```python
from build123d import *

# Parameters (mm, degrees)
BOSS_EXTRUDE1_DEPTH = 2.5
SKETCH3_R           = 4
CUT_EXTRUDE2_DEPTH  = 5


with BuildPart() as part:
    # Sketch1 → Boss-Extrude1 (new, symmetric)
    with BuildSketch(Plane(origin=(0, 0, 0), x_dir=(0, 1, 0), z_dir=(0, 0, 1))):
        Polygon((-56, 9.27), (-56, -9.27), (-50, -9.27), (-50, -12.741071429), (-50, -14.27), (-40, -14.27), (-40, -10.192857143), (-40, -9.27), (40, -9.27), (40, -10.192857143), (40, -14.27), (50, -14.27), (50, -9.27), (56, -9.27), (56, 9.27), (50, 9.27), (50, 14.27), (40, 14.27), (40, 9.27), (-40, 9.27), (-40, 10.192857143), (-40, 14.27), (-50, 14.27), (-50, 12.741071429), (-50, 9.27), align=None)
    extrude(amount=BOSS_EXTRUDE1_DEPTH, both=True)

    # Sketch3 → Cut-Extrude2 (cut)
    with BuildSketch(Plane.XY.offset(2.5)):
        with Locations((0, 40)):
            Circle(SKETCH3_R)
        with Locations((0, -40)):
            Circle(SKETCH3_R)
    extrude(amount=-CUT_EXTRUDE2_DEPTH, mode=Mode.SUBTRACT)


solid = part.part
```
For this review, take the finished solid that the model builds, in its own axes (mm). A direction names the side the tool comes from. Give positions to 0.01 mm unless a question says otherwise; leave off trailing zeros. Loops run counter-clockwise (first coordinate to the right, second up) from the corner with the lowest first, then second, coordinate; pieces in that order, holes last. Notation, with made-up numbers: M -2.5,24.5 L 54.5,24.5 A14 ccw 54.5,37.5 Z; hole C 41.5,19 d1. An arc over 180 degrees is marked long. One line per item, written item: value. Start each with the question number.
Q1. Machinability: for faces 4 (the face through (9.27, 53, 0)), 5 (the face through (-9.27, 53, 0)), 6 (the face through (9.27, -1, 0)), which of the approach directions +Z, -Z, +X, -X, +Y, -Y give a long, thin tool a straight path to every point of the face, cutting with its end or side? Answer none if there is none.
Q2. Clearance check with flat-ended pins moving along their axes: pin 1 Ø2.5 at (y, z) = (13.5, 0) entering from +X; pin 2 Ø2.5 at (x, z) = (-12.5, 0.5) entering from -Y; pin 3 Ø1 at (y, z) = (-23.5, 0) entering from -X. State where each tip first meets the part, or that it passes through.
Q3. Add section B-B (y = 31.5). Give the boundary of the cut face in (x, z), and give its area (3 significant figures).
Q4. Add section A-A (x = 0). Give the boundary of the cut face in (y, z), and give its area (3 significant figures).
Q5. Draft analysis for pull direction Y (two halves, no side actions). For faces 1 (the face through (12, 50, 0)), 2 (the face through (0, -1, -2.5)), 3 (the face through (-12, 40, 0)), state which applies: released by +Y, released by -Y, zero draft, split by the parting line, or undercut.
Q6. For L1, parallel to Y at x = 0, z = -0.45; L2, parallel to Y at x = -12.75, z = -1; L3, parallel to X at y = 51.5, z = -0.95, list the stretches that pass through material, from the lowest coordinate up.
Reply:
1. face 4: +Z, -Z, +X, +Y
1. face 5: +Z, -Z, -X, +Y
1. face 6: +Z, -Z, +X
2. pin 1: x = 9.27
2. pin 2: y = -50
2. pin 3: x = -9.27
3. outline: M -9.27,-2.5 L 9.27,-2.5 L 9.27,2.5 L -9.27,2.5 Z
3. area: 92.7 mm²
4. outline: M -56,-2.5 L -44,-2.5 L -44,2.5 L -56,2.5 Z; M -36,-2.5 L 36,-2.5 L 36,2.5 L -36,2.5 Z; M 44,-2.5 L 56,-2.5 L 56,2.5 L 44,2.5 Z
4. area: 480 mm²
5. face 1: released by +Y
5. face 2: zero draft
5. face 3: undercut
6. L1: -56 to -44, -36 to 36, 44 to 56
6. L2: -50 to -40, 40 to 50
6. L3: -9.27 to 9.27
